Input: part model. Units: mm. Frame: model coordinates. Coordinates: 2 decimals unless noted, no trailing zeros. Write each loop counter-clockwise with the first axis right and the second up, starting at its lowest first coordinate (ties: lowest second). Pieces come first, ordered by that corner, then holes. Notation, with made-up numbers: (58.25, -19) - (103.25, -19) arc R18 ccw to (103.25, -6) - close; hole circle Ø5 at (-10.75, -11). An arc over 180 degrees is marked (long way). Use a Markdown table: item, result. Add a question column.
Q1. Pin query (flat end, axial travel): P1, Ø0.8, axis at x = 0.5, z = 0.5, coming from the -Y side. Return the tip coordinate at first contact, or that it passes through.
Q2. Section query B-B (y = -133.35). Return the cut outline in (x, z), then the cut area to 3 significant figures.
Q3. Material intervals for probe 1 along X at (y, z) = (-152.4, 1.1); probe 2 along Y at (x, z) = (6.35, 0.6); probe 3 along Y at (x, z) = (-6.35, 0.85), sorted ascending. Write a range as from..to.
Q4. Section query C-C (x = -6.35). Return the cut outline in (y, z), then the cut area to 3 significant figures.
Q5. Section query A-A (x = 6.35). Return the cut outline in (y, z), then the cut area to 3 significant figures.
Q6. Section query D-D (y = -114.3). Return the cut outline in (x, z), then the cut area to 3 significant figures.
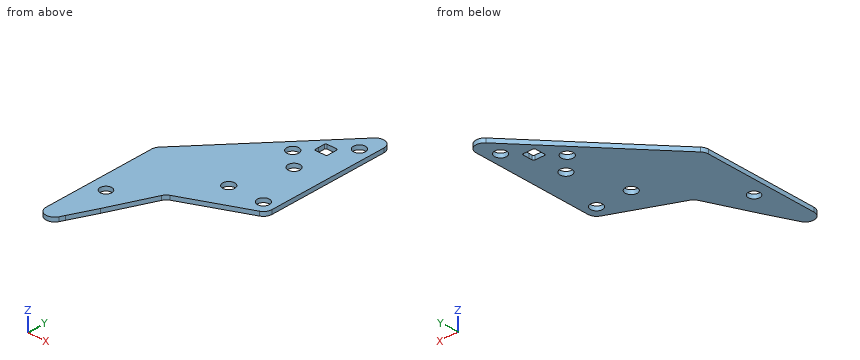
Autodesk Inventor part; units mm, degrees
ref_plane "YZ Plane" through (0, 0, 0) normal (1, 0, 0) x (0, 1, 0)
ref_plane "XZ Plane" through (0, 0, 0) normal (0, 1, 0) x (-1, 0, 0)
ref_plane "XY Plane" through (0, 0, 0) normal (0, 0, 1) x (1, 0, 0)
sketch "Sketch1" plane through (0, 0, 0) normal (0, 0, 1) x (1, 0, 0)
  line L0 (-27.7783, -197.0642) -> (-31.3026, -204.3884)
  line L1 (-31.4232, -201.1242) -> (-27.8989, -193.8)
  line L2 (-27.8989, -193.8) -> (-23.4904, -184.6379)
  line L3 (-23.4904, -184.6379) -> (-28.7106, -195.4868)
  line L4 (-34.7466, -194.1101) -> (-34.7466, -152.2155)
  line L5 (-33.912, -150.07) -> (5.3023, -107.292)
  line L6 (10.8178, -109.4374) -> (10.8178, -153.8408)
  line L7 (8.906, -156.7537) -> (-14.4444, -166.8799)
  line L8 (-16.0666, -168.4681) -> (-23.4904, -184.6379)
  arc A0 (10.8178, -109.4374) -> (5.3023, -107.292) centre (7.6428, -109.4374) ccw
  arc A1 (8.906, -156.7537) -> (10.8178, -153.8408) centre (7.6428, -153.8408) ccw
  arc A2 (-14.4444, -166.8799) -> (-16.0666, -168.4681) centre (-13.1812, -169.7928) ccw
  arc A3 (-34.7466, -194.1101) -> (-28.7106, -195.4868) centre (-31.5716, -194.1101) ccw
  arc A4 (-33.912, -150.07) -> (-34.7466, -152.2155) centre (-31.5716, -152.2155) ccw
  circle A5 centre (6.35, -152.4) radius 2.1844
  circle A6 centre (-6.35, -152.4) radius 2.1844
  circle A7 centre (6.35, -114.3) radius 2.1844
  circle A8 centre (-6.35, -127) radius 2.1844
  circle A9 centre (-29.0224, -176.553) radius 2.0955
  line L9 (2.2749, -122.43) -> (2.2749, -121.1289)
  spline S0 degree 3 poles (2.2749, -121.1289) (2.2749, -120.7564) (2.2756, -120.3847) (2.2775, -119.644) (2.2787, -119.2745) (2.2799, -118.9051) knots 0 0 0 0 0.001117 0.001117 0.002234 0.002234 0.002234 0.002234
  arc A10 (1.78, -122.9249) -> (2.2749, -122.43) centre (1.78, -122.43) ccw
  arc A11 (2.2799, -118.87) -> (1.78, -118.3701) centre (1.78, -118.87) ccw
  spline S1 degree 3 poles (2.2799, -118.9051) (2.2799, -118.8934) (2.2799, -118.8817) (2.2799, -118.87) knots 0 0 0 0 0.000035 0.000035 0.000035 0.000035
  line L10 (1.78, -118.3701) -> (-1.78, -118.3701)
  arc A12 (-1.78, -118.3701) -> (-2.2799, -118.87) centre (-1.78, -118.87) ccw
  spline S2 degree 3 poles (-2.2799, -118.9051) (-2.2787, -119.2745) (-2.2775, -119.644) (-2.2756, -120.3847) (-2.2749, -120.7564) (-2.2749, -121.1289) knots 0.000013 0.000013 0.000013 0.000013 0.001129 0.001129 0.002246 0.002246 0.002246 0.002246
  spline S3 degree 3 poles (-2.2799, -118.87) (-2.2799, -118.8817) (-2.2799, -118.8934) (-2.2799, -118.9051) knots 0 0 0 0 0.000035 0.000035 0.000035 0.000035
  line L11 (-2.2749, -121.1289) -> (-2.2749, -122.43)
  arc A13 (-2.2749, -122.43) -> (-1.78, -122.9249) centre (-1.78, -122.43) ccw
  line L12 (-1.78, -122.9249) -> (1.78, -122.9249)
  circle A14 centre (0, -133.35) radius 2.1844
  point P0 (0, 0)
  point P1 (-34.7466, -208.031)
  dimension "d0" = 1.524
  dimension "d1" = 3.175
  dimension "d2" = 4.191
extrude "Extrusion1" add sketch "Sketch1" along normal blind 1.524
properties part number "back-sled"
Values follow:
| question | item | result |
|---|---|---|
| 1 | P1 | y = -160.57 |
| 2 | outline | (-18.58, 0) - (-2.18, 0) - (-2.18, 1.52) - (-18.58, 1.52) - close; (2.18, 0) - (10.82, 0) - (10.82, 1.52) - (2.18, 1.52) - close |
| 2 | area | 38.2 mm2 |
| 3 | probe 1 | -34.75..-8.53, -4.17..4.17, 8.53..10.82 |
| 3 | probe 2 | -157.86..-154.58, -150.22..-116.48, -112.12..-106.54 |
| 3 | probe 3 | -163.37..-154.58, -150.22..-129.18, -124.82..-120 |
| 4 | outline | (-163.37, 0) - (-154.58, 0) - (-154.58, 1.52) - (-163.37, 1.52) - close; (-150.22, 0) - (-129.18, 0) - (-129.18, 1.52) - (-150.22, 1.52) - close; (-124.82, 0) - (-120, 0) - (-120, 1.52) - (-124.82, 1.52) - close |
| 4 | area | 52.8 mm2 |
| 5 | outline | (-157.86, 0) - (-154.58, 0) - (-154.58, 1.52) - (-157.86, 1.52) - close; (-150.22, 0) - (-116.48, 0) - (-116.48, 1.52) - (-150.22, 1.52) - close; (-112.12, 0) - (-106.54, 0) - (-106.54, 1.52) - (-112.12, 1.52) - close |
| 5 | area | 64.9 mm2 |
| 6 | outline | (-1.12, 0) - (4.17, 0) - (4.17, 1.52) - (-1.12, 1.52) - close; (8.53, 0) - (10.82, 0) - (10.82, 1.52) - (8.53, 1.52) - close |
| 6 | area | 11.5 mm2 |
